Design review of the part built by this model. Coordinates are the model's own, in mm. Round coordinates to 2 decimals unless told otherwise and drop trailing zeros. Order: outer loops, then holes, each group sorted by start corner. A loop starts at its lowest first (then second) coordinate and runs counter-clockwise, first axis right, second up. Notation, with made-up numbers: (-39.75, -17) - (-7.75, -17) arc R22 ccw to (-7.75, 10) - close; hole circle Ø4 at (29.25, -3.75). An arc over 180 degrees is marked (long way). Answer as a JSON object with one key per item and string values. Group by question number.
from build123d import *

# Parameters (mm, degrees)
F0_W     = 150
F0_H     = 100
F1_DEPTH = 12
F2_SIZE2 = 99.99999
F2_SIZE  = 5.99999


# Not quite as in the source:
# - a fillet or chamfer is up to 0.001 mm smaller than in the source, because OpenCascade refuses the exact size


with BuildPart() as f1:
    # F0 (on Top) → F1 (new body)
    with BuildSketch(Plane.XY):
        with Locations((-75, 50)):
            Rectangle(F0_W, F0_H)
    extrude(amount=F1_DEPTH)

    # F2 (size 6 and 100 in the source; OpenCascade refuses exactly that, so slightly less here)
    f2_edges = [f1.edges().sort_by_distance(p)[0] for p in [
        (-75, 0, 12),
        (-75, 0, 0),
    ]]
    f2_side = f1.faces().sort_by_distance((-75, 0, 6))[0]
    chamfer(f2_edges, length=F2_SIZE, length2=F2_SIZE2, reference=f2_side)


solid = f1.part
1. Mouldability with a two-part tool opening along X and no side actions: class faces 1 (the flat face through (-150, 60, 6)), 2 (the flat face through (0, 60, 6)), 3 (the flat face through (-76, 100, 6)) as pulls with the +X half, pulls with the -X half, needs draft (parallel to the pull), parting line crosses it, or undercut.
2. Take a section at C-C, the plane z = 4.5. Give the boundary of the cut face in (x, y), then the cut area to 4 significant figures.
3. Clearance check with flat-ended pins moving along their axes: P1, Ø1, axis at x = -115.5, y = 46.5, coming from the -Z side; P2, Ø5, axis at x = -25.5, z = 6, coming from the -Y side; P3, Ø2, axis at x = -73.5, y = 22.5, coming from the +Z side. State where each tip first meets the part, or that it passes through.
4. Take a section at B-B, the plane y = 52. Give the boundary of the cut face in (x, z).
5. To check wall thickness, follow line 1 (Z direction, x = -83, y = 58); line 2 (Z direction, x = -109.5, y = 16.5). State the ranges of each line that lie inside material, in increasing order. Write a range as from..to.
Response values:
{
 "1": {"face 1": "pulls with the -X half", "face 2": "pulls with the +X half", "face 3": "needs draft"},
 "2": {"outline": "(-150, 25) - (0, 25) - (0, 100) - (-150, 100) - close", "area": "11,250 mm2"},
 "3": {"P1": "z = 3.18", "P2": "y = 0", "P3": "z = 7.41"},
 "4": {"outline": "(-150, 2.88) - (0, 2.88) - (0, 9.12) - (-150, 9.12) - close"},
 "5": {"line 1": "2.52..9.48", "line 2": "5.01..6.99"}
}
